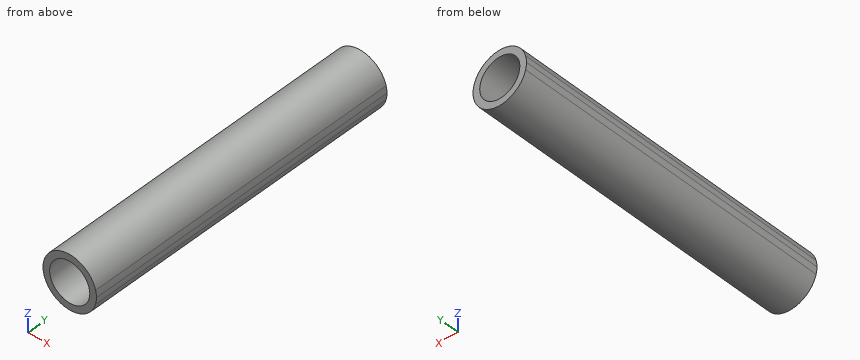
from build123d import *

# Parameters (mm, degrees)
F0_R     = 1.190625
F1_DEPTH = 19.05


with BuildPart() as f1:
    # F0 (on Front) → F1 (new body)
    with BuildSketch(Plane.XZ):
        with BuildLine():
            ThreePointArc((1.5875, 0), (1.574847, 0.200032), (1.53709, 0.396875))
            ThreePointArc((1.53709, 0.396875), (0, 1.5875), (-1.53709, 0.396875))
            ThreePointArc((-1.53709, 0.396875), (-1.574847, 0.200032), (-1.5875, 0))
            ThreePointArc((-1.5875, 0), (-1.574847, -0.200032), (-1.53709, -0.396875))
            ThreePointArc((-1.53709, -0.396875), (0, -1.5875), (1.53709, -0.396875))
            ThreePointArc((1.53709, -0.396875), (1.574847, -0.200032), (1.5875, 0))
        make_face()
        Circle(F0_R, mode=Mode.SUBTRACT)
    extrude(amount=F1_DEPTH)


solid = f1.part
CAD build for the part. Positions are in the model's coordinates, mm. Round coordinates to 2 decimals unless told otherwise and drop trailing zeros. Order: outer loops, then holes, each group sorted by start corner. A loop starts at its lowest first (then second) coordinate and runs counter-clockwise, first axis right, second up. Notation, with made-up numbers: (-39.75, -9) -> (-34.75, -9) arc R8 ccw to (-34.75, 3) -> close; hole circle Ø9 at (-13.5, -18). An arc over 180 degrees is marked (long way). Write item = value, one per line. Start each with the question number.
(1) Cut at C-C, the plane z = 0.8. List the corners of the cut face in (x, y).
(2) Cut at B-B, the plane y = -15.5. List the corners of the cut face in (x, z) (1 decimal).
(3) Pin check, flat tip, straight feed: P1, Ø1, axis at x = 1, y = -7, coming from the -Z side. Stop position of the tip, or through.
(4) Cut at A-A, the plane x = 0. List the corners of the cut face in (y, z).
(5) Probe line 1 (X direction, y = -16.5, z = -0.3); line 2 (Z direction, x = 1, y = -6.75). List the from-to ranges inside material, lowest first. Write a range as [from, to].
Model answer:
q1.outline = (-1.37, -19.05) -> (-0.88, -19.05) -> (-0.88, 0) -> (-1.37, 0) -> close; (0.88, -19.05) -> (1.37, -19.05) -> (1.37, 0) -> (0.88, 0) -> close
q2.outline = (-1.6, 0) arc R1.6 ccw to (-1.5, -0.4) arc R1.6 ccw to (1.5, -0.4) arc R1.6 ccw to (1.6, 0) arc R1.6 ccw to (1.5, 0.4) arc R1.6 ccw to (-1.5, 0.4) arc R1.6 ccw to start; hole circle Ø2.4 at (0, 0)
q3.P1 = -1.51
q4.outline = (-19.05, -1.59) -> (0, -1.59) -> (0, -1.19) -> (-19.05, -1.19) -> close; (-19.05, 1.19) -> (0, 1.19) -> (0, 1.59) -> (-19.05, 1.59) -> close
q5.line_1 = [-1.56, -1.15], [1.15, 1.56]
q5.line_2 = [-1.23, -0.65], [0.65, 1.23]
